```python
from build123d import *

# Parameters (mm, degrees)
F0_W     = 38.1
F0_H     = 38.1
F1_DEPTH = 25.4
F1_TAPER = 3
F2_W     = 71.12
F2_H     = 71.12
F3_DEPTH = 3.175
F3_TAPER = 3


# Not quite as in the source:
# - a feature of the source that left no trace in its solid (it failed there, or was rolled back) is left out


with BuildPart() as f1:
    # F0 (on Top) → F1 (new body)
    with BuildSketch(Plane.XY):
        with Locations((-19.05, 19.05)):
            Rectangle(F0_W, F0_H)
        with Locations((19.05, 19.05)):
            Rectangle(F0_W, F0_H)
        with Locations((-19.05, -19.05)):
            Rectangle(F0_W, F0_H)
        with Locations((19.05, -19.05)):
            Rectangle(F0_W, F0_H)
    extrude(amount=F1_DEPTH, taper=F1_TAPER)

    # F2 (on face) → F3 (join)
    with BuildSketch(Plane.XY.offset(25.4)):
        Rectangle(F2_W, F2_H)
    extrude(amount=F3_DEPTH, taper=F3_TAPER)


solid = f1.part
```
Geometry check sheet. Reference: the model listing, model coordinates, mm. Give positions to 0.01 mm unless a question says otherwise; leave off trailing zeros. Loops run counter-clockwise (first coordinate to the right, second up) from the corner with the lowest first, then second, coordinate; pieces in that order, holes last. Notation, with made-up numbers: M 39,74.5 L 51,74.5 A17 ccw 51,101.5 Z; hole C 34,-30.5 d6. An arc over 180 degrees is marked long. Answer as CSV lines item,"result".
Item 1: Depth check by flat-ended pin: P1, Ø12, axis at x = 21, z = 10.5, coming from the -Y side; P2, Ø6, axis at x = 21.5, z = 25, coming from the +Y side; P3, Ø1, axis at x = -4.5, z = 10, coming from the -Y side. Enter the tip coordinate at first touch or a pass-through.
Values:
P1,"stops at y = -37.86"
P2,"stops at y = 36.95"
P3,"stops at y = -37.6"
Item 2: Material ranges on line 1 (Y direction, x = 17.5, z = 25.25); line 2 (X direction, y = 1.5, z = 25.75); line 3 (X direction, y = 13, z = 19.5), recorded low to high.
Values:
line 1,"y = -36.78 to 36.78"
line 2,"x = -35.54 to 35.54"
line 3,"x = -37.08 to 37.08"
Item 3: Cross-section at D-D on z = 19.75. Record the cut outline in (x, y).
Values:
outline,"M -37.06,-37.06 L 37.06,-37.06 L 37.06,37.06 L -37.06,37.06 Z"
Item 4: Cross-section at A-A on y = 1. Record the cut outline in (x, z) (3 decimals).
Values:
outline,"M -38.1,0 L 38.1,0 L 36.769,25.4 L 35.56,25.4 L 35.394,28.575 L -35.394,28.575 L -35.56,25.4 L -36.769,25.4 Z"
Item 5: Cross-section at C-C on z = 10.5. Record the cut outline in (x, y).
Values:
outline,"M -37.55,-37.55 L 37.55,-37.55 L 37.55,37.55 L -37.55,37.55 Z"
